Autodesk Inventor part; units mm, degrees
ref_plane "YZ Plane" through (0, 0, 0) normal (1, 0, 0) x (0, 1, 0)
ref_plane "XZ Plane" through (0, 0, 0) normal (0, 1, 0) x (-1, 0, 0)
ref_plane "XY Plane" through (0, 0, 0) normal (0, 0, 1) x (1, 0, 0)
ref_plane "Work Plane1" through (-42.5139, 0, 0) normal (0, 0, 1) x (1, 0, 0)
sketch "Sketch1" plane through (-42.5139, 0, 0) normal (0, 0, 1) x (1, 0, 0)
  line L0 (-61.9417, 0) -> (61.9417, 0)
  line L1 (61.9417, 0) -> (61.9417, -14.325)
  line L2 (58.7667, -17.5) -> (-58.7667, -17.5)
  line L3 (-61.9417, -14.325) -> (-61.9417, 0)
  line L4 (-61.9417, -14.325) -> (-61.9417, -7.5)
  line L5 (61.9417, -7.5) -> (61.9417, -14.325)
  line L6 (-75.2, -7.5) -> (75.2, -7.5)
  line L7 (-58.7667, 0) -> (-55.1167, 0)
  line L8 (55.1167, 0) -> (58.7667, 0)
  line L9 (-58.7667, -17.5) -> (-53.0564, -17.5)
  line L10 (53.0564, -17.5) -> (58.7667, -17.5)
  arc A0 (-61.9417, -14.325) -> (-58.7667, -17.5) centre (-58.7667, -14.325) ccw
  arc A1 (58.7667, -17.5) -> (61.9417, -14.325) centre (58.7667, -14.325) ccw
  circle A2 centre (-56.9417, -3.75) radius 1.524
  circle A3 centre (-56.9417, -12.5) radius 1.524
  circle A4 centre (56.9417, -12.5) radius 1.524
  circle A5 centre (56.9417, -3.75) radius 1.524
  line L11 (-43.3353, -7.5) -> (43.3353, -7.5)
  line L12 (43.3353, -7.5) -> (43.3353, -17.5)
  line L13 (43.3353, -17.5) -> (-43.3353, -17.5)
  line L14 (-43.3353, -17.5) -> (-43.3353, -7.5)
  line L15 (-43.3353, -11.5) -> (43.3353, -11.5)
  line L16 (-58.7667, -17.5) -> (-53.0564, -17.5)
  line L17 (-58.7667, -17.5) -> (-53.0564, -17.5)
  line L18 (53.0564, -17.5) -> (58.7667, -17.5)
  line L19 (43.3353, -7.5) -> (53.0564, -17.5)
  line L20 (-53.0564, -17.5) -> (-43.3353, -7.5)
  line L21 (-56.9417, -3.75) -> (56.9417, -3.75) construction
  line L22 (-51.9417, -7.5) -> (-51.9417, -3.175)
  line L23 (51.9417, -3.175) -> (51.9417, -7.5)
  circle A6 centre (-43.2848, -3.75) radius 1.27
  circle A7 centre (-25.9709, -3.75) radius 1.27
  circle A8 centre (-8.657, -3.75) radius 1.27
  circle A9 centre (8.657, -3.75) radius 1.27
  circle A10 centre (25.9709, -3.75) radius 1.27
  circle A11 centre (43.2848, -3.75) radius 1.27
  line L24 (-51.9417, 0) -> (51.9417, 0)
  line L25 (51.9417, 0) -> (51.9417, 7.112)
  line L26 (51.9417, 7.112) -> (-51.9417, 7.112)
  line L27 (-51.9417, 7.112) -> (-51.9417, 0)
  circle A12 centre (-43.2848, 0) radius 1.133
  circle A13 centre (-43.2848, 5) radius 1.133
  line L28 (-44.4178, 5) -> (-44.4178, 0)
  line L29 (-42.1518, 0) -> (-42.1518, 5)
  circle A14 centre (-25.9709, 0) radius 1.133
  circle A15 centre (-25.9709, 5) radius 1.133
  line L30 (-27.1039, 5) -> (-27.1039, 0)
  line L31 (-24.8379, 0) -> (-24.8379, 5)
  circle A16 centre (-8.657, 0) radius 1.133
  circle A17 centre (-8.657, 5) radius 1.133
  line L32 (-9.79, 5) -> (-9.79, 0)
  line L33 (-7.524, 0) -> (-7.524, 5)
  circle A18 centre (8.657, 0) radius 1.133
  circle A19 centre (8.657, 5) radius 1.133
  line L34 (7.524, 5) -> (7.524, 0)
  line L35 (9.79, 0) -> (9.79, 5)
  circle A20 centre (25.9709, 0) radius 1.133
  circle A21 centre (25.9709, 5) radius 1.133
  line L36 (24.8379, 5) -> (24.8379, 0)
  line L37 (27.1039, 0) -> (27.1039, 5)
  circle A22 centre (43.2848, 0) radius 1.133
  circle A23 centre (43.2848, 5) radius 1.133
  line L38 (42.1518, 5) -> (42.1518, 0)
  line L39 (44.4178, 0) -> (44.4178, 5)
  point P0 (42.5139, 0)
  point P1 (0, -3.75)
  point P2 (-27.1039, 0)
  point P3 (7.524, 0)
  point P4 (24.8379, 0)
  point P5 (27.1039, 0)
  point P6 (42.1518, 0)
  point P7 (44.4178, 0)
  point P8 (27.1039, 0)
  point P9 (24.8379, 0)
  point P10 (9.79, 0)
  point P11 (7.524, 0)
  point P12 (-7.524, 0)
  point P13 (-9.79, 0)
  point P14 (-24.8379, 0)
  point P15 (-27.1039, 0)
  point P16 (-42.1518, 0)
  dimension "d1" = 3.175
  dimension "d2" = 3.75
  dimension "d5" = 2.54
  dimension "d6" = 103.8834
  dimension "d10" = 17.3139
  dimension "d15" = 8.657
  dimension "d19" = 86.5695
  dimension "d20" = 8.657
  dimension "d21" = 7.112
  dimension "d22" = 2.266
  dimension "d23" = 2.266
  dimension "d25" = 5
  dimension "d29" = 17.3139
extrude "Extrusion1" add sketch "Sketch1" along normal blind 3.175 contours L0 A12 A14 A16 A18 A20 A22 L1 L6 L3 | L6 L20 L2 A0 L3 | L27 L26 L25 L0 L39 A23 L38 L37 A21 L36 L35 A19 L34 L33 A17 L32 L31 A15 L30 L29 A13 L28 | L6 L12 L15 L14 | L14 L2 L20 | L19 L2 L12 | L6 L1 A1 L2 L19 | L15 L12 L2 L14
fillet "Fillet1" radius 3.175 6 edges at (9.4278, 0, 1.5875) (9.4278, 7.112, 1.5875) (-94.4556, 7.112, 1.5875) (-94.4556, 0, 1.5875) (-104.4556, 0, 1.5875) (19.4278, 0, 1.5875)
equation "\"d10\" = 0.166667 * d6"
equation "\"d20\" = -0.5 * d19 + 0.5 * d6"
equation "\"d23\" = d22"
equation "\"d29\" = d10"
properties part number "servo_mount_2"
Here's how the part is built. I have some questions about the finished solid (model axes, mm). A direction names the side the tool comes from. Round coordinates to 2 decimals unless told otherwise and drop trailing zeros. Write each loop counter-clockwise with the first axis right and the second up, starting at its lowest first coordinate (ties: lowest second). Pieces come first, ordered by that corner, then holes.
Q1. If we section it at A-A on y = -12.5: Write out the boundary of the cut face in (x, z) (3 decimals).
Q2. If we section it at B-B on z = 1.7: Give the number of separate pieces and of enclosed holes in the cut face, plus the area to 3 significant figures.
Q3. If we mould it in two halves opening along X, with no side actions, what happens to faces 1 (the cylindrical face through (10.333, 0.955, 1.61)), 2 (the cylindrical face through (-67.273, -4.131, 1.565)), 3 (the cylindrical face through (-93.5, 6.21, 1.61))? For each: +X half, -X half, draft (parallel to the pull), parting line (faces both ways), or undercut.
Q4. Which directions (+Z, -Z, +X, -X, +Y, -Y) give clear straight access to the entire face, cutting with the end or side of a thin tool? Please do faces 4 (the flat face through (-84.666, 2, 2)), 5 (the flat face through (19.428, -9, 2)).
Q5. Please list where these lines run through material, in increasing order: probe 1 along Y at (x, z) = (-33, 2.1); probe 2 along Y at (x, z) = (-33.5, 1.95); probe 3 along X at (y, z) = (-13, 1.9).
Q6. Will these pins go through, and if not, where does the flat tip stop? P1, Ø1.6, axis at x = -99.5, z = 2, coming from the +Y side; P2, Ø4, axis at x = 14.43, y = -12.5, coming from the +Z side (3 decimals); P3, Ø0.8, axis at y = 3.5, z = 2, coming from the -X side; P4, Ø1, axis at y = 1, z = 1, coming from the +X side.
Answer below:
1. outline: (-104.456, 0) - (-100.98, 0) - (-100.98, 3.175) - (-104.456, 3.175) - close; (-97.932, 0) - (12.904, 0) - (12.904, 3.175) - (-97.932, 3.175) - close; (15.952, 0) - (19.428, 0) - (19.428, 3.175) - (15.952, 3.175) - close
2. separate pieces: 1
2. enclosed holes: 16
2. area: 2,750 mm2
3. face 1: +X half
3. face 2: undercut
3. face 3: -X half
4. face 4: +Z, -Z
4. face 5: +Z, -Z, +X, +Y, -Y
5. probe 1: y = -17.5 to -4.69, -2.81 to -0.74, 5.74 to 7.11
5. probe 2: y = -17.5 to -4.97, -2.53 to -1.08, 6.08 to 7.11
5. probe 3: x = -104.46 to -100.9, -98.02 to 12.99, 15.87 to 19.43
6. P1: stops at y = 0
6. P2: stops at z = 3.175
6. P3: stops at x = -94.46
6. P4: stops at x = 10.89
